Can you work these out from the model? Positions are in its coordinate system, mm. Face numbers are marked on the shaded views. A direction names the side the tool comes from. Round coordinates to 2 decimals unless told otherwise and drop trailing zeros. Loops run counter-clockwise (first coordinate to the right, second up) from the corner with the lowest first, then second, coordinate; pieces in that order, holes last. Notation, with made-up numbers: (11, 19.5) -> (43, 19.5) arc R25 ccw to (43, 50.5) -> close; hole circle Ø6 at (63, -11). An arc over 180 degrees is marked (long way). Answer as a JSON object with one key per item and string values.
```python
from build123d import *

# Parameters (mm, degrees)
BASPROSKE_W              = 12.7
BASPROSKE_H              = 31.115
TOOTHCUT_DEPTH           = 46.799306217
TEETHCUTS_COUNT          = 47
TEETHCUTS_ANGLE          = 352.340425532
BORSKE_R                 = 1.5875
BORE_DEPTH               = 50.8000508
CUT_EXTRUDE2_DEPTH       = 46.794769115
BOSS_EXTRUDE1_DEPTH      = 19.05
BOSS_EXTRUDE1_DEPTH_BACK = 12.7
SKETCH2_W                = 19.05
SKETCH2_H                = 3.175
SKETCH4_W                = 19.05
SKETCH4_H                = 3.175
BOSS_EXTRUDE2_DEPTH      = 12.7
F_1_4_CLEARANCE_HOLE1_D  = 6.7564


with BuildPart() as part:
    # BasProSke → Base-Revolve (revolve)
    with BuildSketch(Plane(origin=(0, 0, 0), x_dir=(1, 0, 0), z_dir=(0, 1, 0)), mode=Mode.PRIVATE) as base_revolve_sk:
        with Locations((6.35, 15.5575)):
            Rectangle(BASPROSKE_W, BASPROSKE_H)
    revolve(base_revolve_sk.sketch.rotate(Axis((-10, 0, 0), (1, 0, 0)), 180), axis=Axis((-10, 0, 0), (1, 0, 0)))

    # TooCutSke → ToothCut (cut, through all)
    with BuildSketch(Plane(origin=(0, 0, 0), x_dir=(0, 0, -1), z_dir=(1, 0, 0))):
        with BuildLine():
            ThreePointArc((0.567219539, 28.264509018), (0, 28.2702), (-0.567219539, 28.264509018))
            ThreePointArc((-0.567219539, 28.264509018), (-1.041703705, 29.715512743), (-1.697480705, 31.094100267))
            ThreePointArc((-1.697480705, 31.094100267), (0, 31.1404), (1.697480705, 31.094100267))
            ThreePointArc((1.697480705, 31.094100267), (1.041703705, 29.715512743), (0.567219539, 28.264509018))
        make_face()
    toothcut = extrude(amount=TOOTHCUT_DEPTH, mode=Mode.SUBTRACT)

    # TeethCuts: ToothCut ×47 about axis
    teethcuts_axis = Axis((-10, 0, 0), (1, 0, 0))
    for i in range(1, TEETHCUTS_COUNT):
        add(toothcut.rotate(teethcuts_axis, i * TEETHCUTS_ANGLE / (TEETHCUTS_COUNT - 1)), mode=Mode.SUBTRACT)

    # BorSke → Bore (cut, symmetric)
    with BuildSketch(Plane(origin=(0, 0, 0), x_dir=(0, 0, -1), z_dir=(1, 0, 0))):
        with Locations(Location((0, 0, 0), (0, 0, 180))):
            Circle(BORSKE_R)
    extrude(amount=BORE_DEPTH, both=True, mode=Mode.SUBTRACT)

    # Sketch1 → Cut-Extrude2 (cut, through all)
    with BuildSketch(Plane(origin=(12.7, 0, 0), x_dir=(0, 0, -1), z_dir=(1, 0, 0))):
        with BuildLine():
            Line((28.868706313, -11.6078), (-28.868706313, -11.6078))
            ThreePointArc((-28.868706313, -11.6078), (0, 31.115), (28.868706313, -11.6078))
        make_face()
    extrude(amount=-CUT_EXTRUDE2_DEPTH, mode=Mode.SUBTRACT)

    # Sketch2 → Boss-Extrude1 (add, two sides: drawn at the far end of the back side and taken through both)
    with BuildSketch(Plane.ZY.offset(-BOSS_EXTRUDE1_DEPTH_BACK)):
        with Locations((0, -13.1953)):
            Rectangle(SKETCH2_W, SKETCH2_H)
    extrude(amount=BOSS_EXTRUDE1_DEPTH + BOSS_EXTRUDE1_DEPTH_BACK)

    # Sketch4 → Boss-Extrude2 (add)
    with BuildSketch(Plane(origin=(12.7, 0, 0), x_dir=(0, 0, -1), z_dir=(1, 0, 0))):
        with Locations((0, -13.1953)):
            Rectangle(SKETCH4_W, SKETCH4_H)
    extrude(amount=BOSS_EXTRUDE2_DEPTH)

    # 1/4 Clearance Hole1 (through all)
    with Locations(Plane(origin=(19.05, -11.6078, 0), x_dir=(0, 0, 1), z_dir=(0, 1, 0))):
        with Locations((0, 0), (0, -25.4)):
            Hole(F_1_4_CLEARANCE_HOLE1_D / 2)


solid = part.part
```
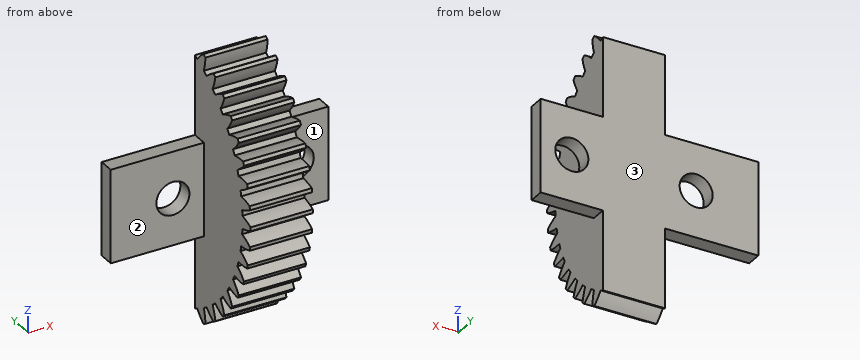
Q1. I want a section at C-C, the plane y = -16.5. Write out the boundary of the cut face in (x, z), then the cut area to 3 significant figures.
Determined:
{"outline": "(0, -24.21) -> (12.7, -24.21) -> (12.7, 24.21) -> (0, 24.21) -> close", "area": "615 mm²"}
Q2. If I drill on L1, parallel to X at y = -13.35, z = 0; L2, parallel to Z at x = 11, y = -30.25; L3, parallel to X at y = -13.5, z = -1, over which ranges is the centre line in solid material (lowest first)? Write a range as [from, to].
Determined:
{"L1": "[-19.05, -9.73], [-2.97, 15.67], [22.43, 25.4]", "L2": "[-4.69, -3.37], [-0.76, 0.76], [3.37, 4.69]", "L3": "[-19.05, -9.58], [-3.12, 15.82], [22.28, 25.4]"}
Q3. I'm going to push flat-ended pins straight in: pin 1 (1.6 mm diameter, centred on x = -10, y = -12.5, fed in from +Z) (3 decimals); pin 2 (4 mm diameter, centred on x = 3.5, y = -17.5, fed in from +Z); pin 3 (1.5 mm diameter, centred on y = -17.5, z = 21.5, fed in from +X); pin 4 (10 mm diameter, centred on x = -12.5, z = 12.5, fed in from +Y). Where does each tip first touch, or does it pass through?
Determined:
{"pin 1": "z = 9.525", "pin 2": "z = 25.28", "pin 3": "x = 12.7", "pin 4": "y = -11.61"}
Q4. I want a section at B-B, the plane x = 20. Write out the boundary of the cut face in (y, z) (3 decimals), then the cut area to 3 significant figures.
Determined:
{"outline": "(-14.783, -9.525) -> (-11.608, -9.525) -> (-11.608, -3.242) -> (-14.783, -3.242) -> close; (-14.783, 3.242) -> (-11.608, 3.242) -> (-11.608, 9.525) -> (-14.783, 9.525) -> close", "area": "39.9 mm²"}
Q5. I want a section at A-A, the plane x = -6.35. Write out the boundary of the cut face in (y, z) (3 decimals), then the cut area to 3 significant figures.
Determined:
{"outline": "(-14.783, -9.525) -> (-11.608, -9.525) -> (-11.608, -3.378) -> (-14.783, -3.378) -> close; (-14.783, 3.378) -> (-11.608, 3.378) -> (-11.608, 9.525) -> (-14.783, 9.525) -> close", "area": "39.0 mm²"}
Q6. On a 3-axis mill with a long thin cutter (end or side, diameter ignored), from which of +Z, -Z, +X, -X, +Y, -Y can I reach the whole of each face in a straight line? I mean the marked faces 1, 2 and 3. Say none if no direction works.
Determined:
{"face 1": "+Z, -Z, +X, -Y", "face 2": "+Z, -Z, -X, -Y", "face 3": "+Z, -Z, +X, -X, +Y"}
Q7. I want a section at D-D, the plane x = -11. Write out the boundary of the cut face in (y, z) (3 decimals).
Determined:
{"outline": "(-14.783, -9.525) -> (-11.608, -9.525) -> (-11.608, 9.525) -> (-14.783, 9.525) -> close"}
